from build123d import *

# Parameters (mm, degrees)
BOSS_EXTRUDE1_DEPTH            = 32.512
SKETCH2_R                      = 5.9436
BOSS_EXTRUDE2_DEPTH            = 1.27
SKETCH3_R                      = 5.9436
BOSS_EXTRUDE3_DEPTH            = 1.27
BOSS_EXTRUDE4_DEPTH            = 65.8368
BOSS_EXTRUDE5_DEPTH            = 12.4206
SKETCH6_R                      = 5.9436
BOSS_EXTRUDE6_DEPTH            = 1.27
BOSS_EXTRUDE7_DEPTH            = 12.4206
F_7_0_201_DIAMETER_HOLE1_D     = 5.1054
F_7_0_201_DIAMETER_HOLE1_DEPTH = 127


with BuildPart() as part:
    # Sketch1 → Boss-Extrude1 (new body)
    with BuildSketch(Plane.XY.offset(-17.2974)):
        with BuildLine():
            Line((-4.187390656, 5.447226632), (-6.811131972, 0.902773368))
            ThreePointArc((-6.811131972, 0.902773368), (-6.8707, 0), (-6.811131972, -0.902773368))
            Line((-6.811131972, -0.902773368), (-4.187390656, -5.447226632))
            ThreePointArc((-4.187390656, -5.447226632), (-3.43535, -5.950200742), (-2.623741315, -6.35))
            Line((-2.623741315, -6.35), (2.623741315, -6.35))
            ThreePointArc((2.623741315, -6.35), (3.43535, -5.950200742), (4.187390656, -5.447226632))
            Line((4.187390656, -5.447226632), (6.811131972, -0.902773368))
            ThreePointArc((6.811131972, -0.902773368), (6.8707, 0), (6.811131972, 0.902773368))
            Line((6.811131972, 0.902773368), (4.187390656, 5.447226632))
            ThreePointArc((4.187390656, 5.447226632), (3.43535, 5.950200742), (2.623741315, 6.35))
            Line((2.623741315, 6.35), (-2.623741315, 6.35))
            ThreePointArc((-2.623741315, 6.35), (-3.43535, 5.950200742), (-4.187390656, 5.447226632))
        make_face()
    extrude(amount=-BOSS_EXTRUDE1_DEPTH)

    # Sketch2 → Boss-Extrude2 (add)
    with BuildSketch(Plane(origin=(0, 0, -49.8094), x_dir=(-1, 0, 0), z_dir=(0, 0, -1))):
        Circle(SKETCH2_R)
    extrude(amount=BOSS_EXTRUDE2_DEPTH)

    # Sketch3 → Boss-Extrude3 (add)
    with BuildSketch(Plane.XY.offset(-17.2974)):
        Circle(SKETCH3_R)
    extrude(amount=BOSS_EXTRUDE3_DEPTH)

    # Sketch4 → Boss-Extrude4 (add)
    with BuildSketch(Plane(origin=(0, 0, -16.0274), x_dir=(-1, 0, 0), z_dir=(0, 0, -1))):
        with BuildLine():
            Line((2.623741315, 6.35), (-2.623741315, 6.35))
            ThreePointArc((-2.623741315, 6.35), (-3.43535, 5.950200742), (-4.187390656, 5.447226632))
            Line((-4.187390656, 5.447226632), (-6.811131972, 0.902773368))
            ThreePointArc((-6.811131972, 0.902773368), (-6.8707, 0), (-6.811131972, -0.902773368))
            Line((-6.811131972, -0.902773368), (-4.187390656, -5.447226632))
            ThreePointArc((-4.187390656, -5.447226632), (-3.43535, -5.950200742), (-2.623741315, -6.35))
            Line((-2.623741315, -6.35), (2.623741315, -6.35))
            ThreePointArc((2.623741315, -6.35), (3.43535, -5.950200742), (4.187390656, -5.447226632))
            Line((4.187390656, -5.447226632), (6.811131972, -0.902773368))
            ThreePointArc((6.811131972, -0.902773368), (6.8707, 0), (6.811131972, 0.902773368))
            Line((6.811131972, 0.902773368), (4.187390656, 5.447226632))
            ThreePointArc((4.187390656, 5.447226632), (3.43535, 5.950200742), (2.623741315, 6.35))
        make_face()
    extrude(amount=-BOSS_EXTRUDE4_DEPTH)

    # Sketch5 → Boss-Extrude5 (add)
    with BuildSketch(Plane.XY.offset(-51.0794)):
        with BuildLine():
            Line((-4.187390656, 5.447226632), (-6.811131972, 0.902773368))
            ThreePointArc((-6.811131972, 0.902773368), (-6.8707, 0), (-6.811131972, -0.902773368))
            Line((-6.811131972, -0.902773368), (-4.187390656, -5.447226632))
            ThreePointArc((-4.187390656, -5.447226632), (-3.43535, -5.950200742), (-2.623741315, -6.35))
            Line((-2.623741315, -6.35), (2.623741315, -6.35))
            ThreePointArc((2.623741315, -6.35), (3.43535, -5.950200742), (4.187390656, -5.447226632))
            Line((4.187390656, -5.447226632), (6.811131972, -0.902773368))
            ThreePointArc((6.811131972, -0.902773368), (6.8707, 0), (6.811131972, 0.902773368))
            Line((6.811131972, 0.902773368), (4.187390656, 5.447226632))
            ThreePointArc((4.187390656, 5.447226632), (3.43535, 5.950200742), (2.623741315, 6.35))
            Line((2.623741315, 6.35), (-2.623741315, 6.35))
            ThreePointArc((-2.623741315, 6.35), (-3.43535, 5.950200742), (-4.187390656, 5.447226632))
        make_face()
    extrude(amount=-BOSS_EXTRUDE5_DEPTH)

    # Sketch6 → Boss-Extrude6 (add)
    with BuildSketch(Plane.XY.offset(49.8094)):
        Circle(SKETCH6_R)
    extrude(amount=BOSS_EXTRUDE6_DEPTH)

    # Sketch7 → Boss-Extrude7 (add)
    with BuildSketch(Plane(origin=(0, 0, 51.0794), x_dir=(-1, 0, 0), z_dir=(0, 0, -1))):
        with BuildLine():
            Line((6.811131972, 0.902773368), (4.187390656, 5.447226632))
            ThreePointArc((4.187390656, 5.447226632), (3.43535, 5.950200742), (2.623741315, 6.35))
            Line((2.623741315, 6.35), (-2.623741315, 6.35))
            ThreePointArc((-2.623741315, 6.35), (-3.43535, 5.950200742), (-4.187390656, 5.447226632))
            Line((-4.187390656, 5.447226632), (-6.811131972, 0.902773368))
            ThreePointArc((-6.811131972, 0.902773368), (-6.8707, 0), (-6.811131972, -0.902773368))
            Line((-6.811131972, -0.902773368), (-4.187390656, -5.447226632))
            ThreePointArc((-4.187390656, -5.447226632), (-3.43535, -5.950200742), (-2.623741315, -6.35))
            Line((-2.623741315, -6.35), (2.623741315, -6.35))
            ThreePointArc((2.623741315, -6.35), (3.43535, -5.950200742), (4.187390656, -5.447226632))
            Line((4.187390656, -5.447226632), (6.811131972, -0.902773368))
            ThreePointArc((6.811131972, -0.902773368), (6.8707, 0), (6.811131972, 0.902773368))
        make_face()
    extrude(amount=-BOSS_EXTRUDE7_DEPTH)

    # #7 (0.201) Diameter Hole1
    with Locations(Plane(origin=(0, 0, -63.5), x_dir=(-1, 0, 0), z_dir=(0, 0, -1))):
        with Locations((0, 0)):
            Hole(F_7_0_201_DIAMETER_HOLE1_D / 2, depth=F_7_0_201_DIAMETER_HOLE1_DEPTH)


solid = part.part
Source: CAD feature listing. Evaluate the final solid. Frame: model axes, mm. A direction names the side the tool comes from. Give positions to 0.01 mm unless a question says otherwise; leave off trailing zeros. Order: outer loops, then holes, each group sorted by start corner. A loop starts at its lowest first (then second) coordinate and runs counter-clockwise, first axis right, second up. Notation, with made-up numbers: (78, 28.5) -> (103, 28.5) arc R22 ccw to (103, 66.5) -> close; hole circle Ø4 at (5.25, -18.75). An arc over 180 degrees is marked (long way). Write item = value, one per line.
Q1. Material intervals for line 1 (Z direction, x = 6.25, y = 0.5); line 2 (Y direction, x = 0, z = 7.5); line 3 (Y direction, x = 0.5, z = -31), sorted ascending. Write a range as from..to.
Data:
line_1 = -63.5..-51.08, -49.81..-17.3, -16.03..49.81, 51.08..63.5
line_2 = -6.35..-2.55, 2.55..6.35
line_3 = -6.35..-2.5, 2.5..6.35
Q2. Pin query (flat end, axial travel): pin 1 (1 mm diameter, centred on y = -2, z = 21.5, fed in from -X); pin 2 (1 mm diameter, centred on y = -4, z = 12, fed in from +X); pin 3 (3 mm diameter, centred on x = 0, y = 0, fed in from -Z); pin 4 (2 mm diameter, centred on x = 4, z = 37, fed in from -Y). Return the tip coordinate at first contact, or that it passes through.
Data:
pin_1 = -6.47
pin_2 = 5.31
pin_3 = through
pin_4 = -6.18
Q3. Set-up query: faces 1 (the face through (2, -6, -16.027)), 2 (the face through (0, 6.35, 16)). Return all of +Z, -Z, +X, -X, +Y, -Y with unobstructed straight access to the full face (end or side cutting, diameter ignored); none if empty.
Data:
face_1 = none
face_2 = +Z, -Z, +X, -X, +Y
Q4. Cut plane C-C, the plane y = 3.75. Output: boundary loops of the cut face in (x, z), and give its area (3 significant figures).
Data:
outline = (-5.17, -63.5) -> (5.17, -63.5) -> (5.17, -51.08) -> (4.61, -51.08) -> (4.61, -49.81) -> (5.17, -49.81) -> (5.17, -17.3) -> (4.61, -17.3) -> (4.61, -16.03) -> (5.17, -16.03) -> (5.17, 49.81) -> (4.61, 49.81) -> (4.61, 51.08) -> (5.17, 51.08) -> (5.17, 63.5) -> (-5.17, 63.5) -> (-5.17, 51.08) -> (-4.61, 51.08) -> (-4.61, 49.81) -> (-5.17, 49.81) -> (-5.17, -16.03) -> (-4.61, -16.03) -> (-4.61, -17.3) -> (-5.17, -17.3) -> (-5.17, -49.81) -> (-4.61, -49.81) -> (-4.61, -51.08) -> (-5.17, -51.08) -> close
area = 1,310 mm^2
Q5. Pull-direction query (Z, two-part tool) for faces 3 (the face through (0, -3, 63.5)), 4 (the face through (5.52, 3.14, -33.33)), 5 (the face through (-5.669, 1.785, -50.436)); classes: released by +Z, released by -Z, zero draft, split by the parting line, or undercut.
Data:
face_3 = released by +Z
face_4 = zero draft
face_5 = undercut
Q6. Cut plane A-A, the plane z = -36.5. Output: boundary loops of the cut face in (x, y).
Data:
outline = (-6.81, -0.9) -> (-4.19, -5.45) arc R6.87 ccw to (-2.62, -6.35) -> (2.62, -6.35) arc R6.87 ccw to (4.19, -5.45) -> (6.81, -0.9) arc R6.87 ccw to (6.81, 0.9) -> (4.19, 5.45) arc R6.87 ccw to (2.62, 6.35) -> (-2.62, 6.35) arc R6.87 ccw to (-4.19, 5.45) -> (-6.81, 0.9) arc R6.87 ccw to start; hole circle Ø5.11 at (0, 0)
